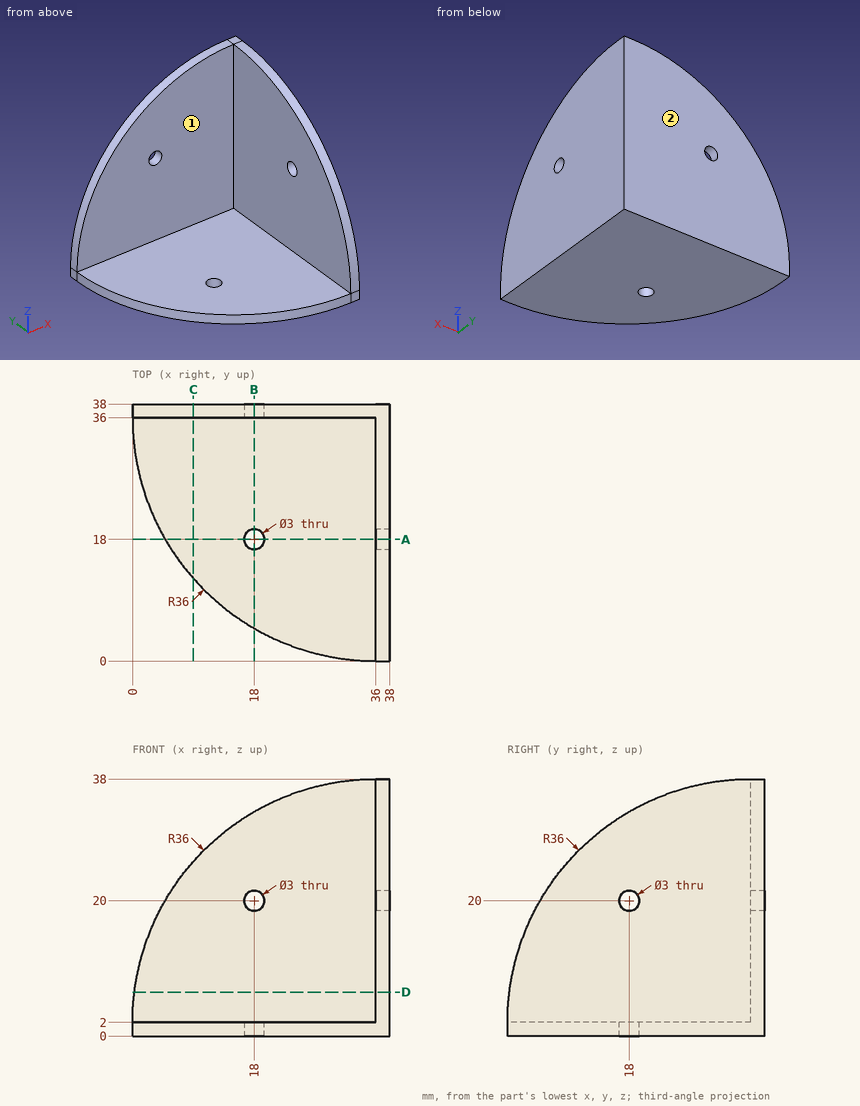
Design review of the part shown in the three views and the two pictorial views. Dimensions are in mm from the part's minimum x, y and z. A direction names the side the tool comes from. Round coordinates to 2 decimals unless told otherwise and drop trailing zeros. Order: outer loops, then holes, each group sorted by start corner. A loop starts at its lowest first (then second) coordinate and runs counter-clockwise, first axis right, second up. Notation, with made-up numbers: (74.25, 35) - (119.25, 35) arc R20 ccw to (119.25, 74) - close; hole circle Ø8 at (38, 54). An arc over 180 degrees is marked (long way). One line per question, with ' | ' between items.
Item 1: Wall thickness on line 1 (Y direction, x = 26, z = 35.5); line 2 (X direction, y = 37.2, z = 20): over which ranges is each line inside the solid? List them lowest first. Write a range as [from, to].
Checks:
line 1: [36, 38] | line 2: [4.82, 16.5], [19.5, 38]
Item 2: For P1, Ø4, axis at y = 18, z = 20, coming from the -X side; P2, Ø6, axis at x = 7, y = 14.5, coming from the +Z side; P3, Ø1, axis at x = 22.5, z = 29, coming from the -Y side; P4, Ø2.5, axis at x = 18, z = 20, coming from the -Y side, all flat-tipped, find the tip position at first contact; note any pin that passes through.
Checks:
P1: x = 36 | P2: z = 2 | P3: y = 36 | P4: through
Item 3: Take a section at A-A, the plane y = 18. Write out the cut boundary in (x, z), then the cut area to 3 significant figures.
Checks:
outline: (4.82, 0) - (16.5, 0) - (16.5, 2) - (4.82, 2) - close; (19.5, 0) - (38, 0) - (38, 18.5) - (36, 18.5) - (36, 2) - (19.5, 2) - close; (36, 21.5) - (38, 21.5) - (38, 33.18) - (36, 33.18) - close | area: 117 mm²
Item 4: Take a section at C-C, the plane x = 9. Write out the cut boundary in (y, z).
Checks:
outline: (12.19, 0) - (38, 0) - (38, 25.81) - (36, 25.81) - (36, 2) - (12.19, 2) - close
Item 5: Machinability: for the marked faces 1 and 2, which of the approach directions +Z, -Z, +X, -X, +Y, -Y give a long, thin tool a straight path to every point of the face, cutting with its end or side? Answer none if there is none.
Checks:
face 1: +Z, -X, -Y | face 2: +Z, -Z, +X, -X, +Y
Item 6: Take a section at D-D, the plane z = 6.5. Write out the cut boundary in (x, y), then the cut area to 3 significant figures.
Checks:
outline: (0.28, 36) - (36, 36) - (36, 0.28) - (38, 0.28) - (38, 38) - (0.28, 38) - close | area: 147 mm²
